from build123d import *

# Parameters (mm, degrees)
F1_DEPTH = 25.4
F2_R     = 5.08
F3_R     = 2.54
F4_DEPTH = 25.4
F5_R     = 2.54
F6_DEPTH = 25.4


with BuildPart() as f1:
    # F0 (on Front) → F1 (new body)
    with BuildSketch(Plane.XZ):
        with BuildLine():
            Line((-12.425265, 4.646856), (-12.425265, 10.895256))
            Line((-12.425265, 10.895256), (-14.635065, 10.895256))
            Line((-14.635065, 10.895256), (-14.635065, -10.288344))
            Line((-14.635065, -10.288344), (-14.635065, -35.688344))
            Line((-14.635065, -35.688344), (-12.425265, -35.688344))
            Line((-12.425265, -35.688344), (-12.425265, -29.439944))
            Line((-12.425265, -29.439944), (-12.425265, -28.48251))
            ThreePointArc((-12.425265, -28.48251), (-11.068052, -28.054224), (-9.941773, -28.924254))
            Line((-9.941773, -28.924254), (-9.941773, -31.308309))
            ThreePointArc((-9.941773, -31.308309), (-9.196233, -32.05385), (-8.450692, -31.308309))
            Line((-8.450692, -31.308309), (-8.450692, -18.884778))
            ThreePointArc((-8.450692, -18.884778), (-9.196233, -18.139237), (-9.941773, -18.884778))
            Line((-9.941773, -18.884778), (-9.941773, -21.268833))
            ThreePointArc((-9.941773, -21.268833), (-11.068052, -22.138863), (-12.425265, -21.710577))
            Line((-12.425265, -21.710577), (-12.425265, -20.753144))
            Line((-12.425265, -20.753144), (-12.425265, -14.504744))
            Line((-12.425265, -14.504744), (-12.425265, -10.288344))
            Line((-12.425265, -10.288344), (-12.425265, -4.039944))
            Line((-12.425265, -4.039944), (-12.425265, -3.08251))
            ThreePointArc((-12.425265, -3.08251), (-11.068052, -2.654224), (-9.941773, -3.524254))
            Line((-9.941773, -3.524254), (-9.941773, -5.908309))
            ThreePointArc((-9.941773, -5.908309), (-9.196233, -6.65385), (-8.450692, -5.908309))
            Line((-8.450692, -5.908309), (-8.450692, 6.515222))
            ThreePointArc((-8.450692, 6.515222), (-9.196233, 7.260763), (-9.941773, 6.515222))
            Line((-9.941773, 6.515222), (-9.941773, 4.131167))
            ThreePointArc((-9.941773, 4.131167), (-11.068052, 3.261137), (-12.425265, 3.689423))
            Line((-12.425265, 3.689423), (-12.425265, 4.646856))
        make_face()
    extrude(amount=-F1_DEPTH)

    # F2
    f2_edges = [f1.edges().sort_by_distance(p)[0] for p in [
        (-13.530165, 25.4, -35.688344),
        (-13.530165, 0, -35.688344),
        (-13.530165, 25.4, 10.895256),
        (-13.530165, 0, 10.895256),
    ]]
    fillet(f2_edges, radius=F2_R)

    # F3 (on face) → F4 (cut)
    with BuildSketch(Plane.YZ.offset(-8.450692)):
        with Locations((12.7, 0)):
            Circle(F3_R)
    extrude(amount=-F4_DEPTH, mode=Mode.SUBTRACT)

    # F5 (on face) → F6 (cut)
    with BuildSketch(Plane.YZ.offset(-8.450692)):
        with Locations((12.7, -25.096544)):
            Circle(F5_R)
    extrude(amount=-F6_DEPTH, mode=Mode.SUBTRACT)


solid = f1.part
Can you work these out from the model? Positions are in its coordinate system, mm. A direction names the side the tool comes from. Give positions to 0.01 mm unless a question says otherwise; leave off trailing zeros. Loops run counter-clockwise (first coordinate to the right, second up) from the corner with the lowest first, then second, coordinate; pieces in that order, holes last. Notation, with made-up numbers: (8, -21.5) -> (33, -21.5) arc R17 ccw to (33, -9.5) -> close; hole circle Ø11 at (85.5, 89.25). An arc over 180 degrees is marked (long way). Use one line per item in the form item = value.
1) If we section it at A-A (z = 0): Please give me the cut outline in (x, y), plus the area to 3 significant figures.
Answers:
outline = (-14.64, 0) -> (-8.45, 0) -> (-8.45, 10.16) -> (-14.64, 10.16) -> close; (-14.64, 15.24) -> (-8.45, 15.24) -> (-8.45, 25.4) -> (-14.64, 25.4) -> close
area = 126 mm²
2) We'd pull the mould along Y, two halves only. Please class faces 1 (the face through (-9.942, 13, -30)), 2 (the face through (-11.5, 10.684, -1.546)), 3 (the face through (-13.51, 23.87, -34.24)): released by +Y, released by -Y, zero draft, split by the parting line, or undercut.
Answers:
face_1 = zero draft
face_2 = undercut
face_3 = released by +Y
3) If we section it at B-B (x = -9.5): Please give me the cut outline in (y, z).
Answers:
outline = (0, -31.99) -> (25.4, -31.99) -> (25.4, -18.2) -> (0, -18.2) -> close; (0, -6.59) -> (25.4, -6.59) -> (25.4, 7.2) -> (0, 7.2) -> close; hole circle Ø5.08 at (12.7, -25.1); hole circle Ø5.08 at (12.7, 0)
4) Will these pins go through, and if not, where does the flat tip stop? pin 1 (4.5 mm diameter, centred on y = 12.7, z = 0, fed in from -X); pin 2 (1.5 mm diameter, centred on x = -9.5, y = 17.5, fed in from +Z).
Answers:
pin_1 = through
pin_2 = 7.26
5) If we section it at D-D (y = 8): Please give me the cut outline in (x, z).
Answers:
outline = (-14.64, -35.69) -> (-12.43, -35.69) -> (-12.43, -28.48) arc R1.54 cw to (-9.94, -28.92) -> (-9.94, -31.31) arc R0.75 ccw to (-8.45, -31.31) -> (-8.45, -18.88) arc R0.75 ccw to (-9.94, -18.88) -> (-9.94, -21.27) arc R1.54 cw to (-12.43, -21.71) -> (-12.43, -3.08) arc R1.54 cw to (-9.94, -3.52) -> (-9.94, -5.91) arc R0.75 ccw to (-8.45, -5.91) -> (-8.45, 6.52) arc R0.75 ccw to (-9.94, 6.52) -> (-9.94, 4.13) arc R1.54 cw to (-12.43, 3.69) -> (-12.43, 10.9) -> (-14.64, 10.9) -> close
6) For faces 4 (the face through (-12.425, 13, 7)), 5 (the face through (-13.55, 1.53, 9.45)), 6 (the face through (-9.213, 12.522, -6.654)), which set-ups out of +Z, -Z, +X, -X, +Y, -Y let a thin tool reach every point of the face, with its end or its side?
Answers:
face_4 = +Z, +Y, -Y
face_5 = +Z, -X, -Y
face_6 = +Y, -Y
7) If we section it at C-C (y = 12.7): Please give me the cut outline in (x, z), plus the area to 3 significant figures.
Answers:
outline = (-14.64, -35.69) -> (-12.43, -35.69) -> (-12.43, -28.48) arc R1.54 cw to (-9.94, -28.92) -> (-9.94, -31.31) arc R0.75 ccw to (-8.45, -31.31) -> (-8.45, -27.64) -> (-14.64, -27.64) -> close; (-14.64, -22.56) -> (-8.45, -22.56) -> (-8.45, -18.88) arc R0.75 ccw to (-9.94, -18.88) -> (-9.94, -21.27) arc R1.54 cw to (-12.43, -21.71) -> (-12.43, -3.08) arc R1.54 cw to (-9.94, -3.52) -> (-9.94, -5.91) arc R0.75 ccw to (-8.45, -5.91) -> (-8.45, -2.54) -> (-14.64, -2.54) -> close; (-14.64, 2.54) -> (-8.45, 2.54) -> (-8.45, 6.52) arc R0.75 ccw to (-9.94, 6.52) -> (-9.94, 4.13) arc R1.54 cw to (-12.43, 3.69) -> (-12.43, 10.9) -> (-14.64, 10.9) -> close
area = 112 mm²
8) I need wall thicknesses on line 1 along X through (y, z) = (21.75, -30.5); line 2 along Y through (x, z) = (-12.75, 6); line 3 along Z through (x, y) = (-10, 12.7). Which ranges of each line are inside material? Lowest first, please.
Answers:
line_1 = -14.64 to -12.43, -9.94 to -8.45
line_2 = 0 to 25.4
line_3 = -28.81 to -27.64, -22.56 to -21.38, -3.41 to -2.54, 2.54 to 4.02
